Part model, mm, in its own coordinate system. Face numbers are marked on the shaded views. A direction names the side the tool comes from. Coordinates: 2 decimals unless noted, no trailing zeros. Order: outer loops, then holes, each group sorted by start corner. A loop starts at its lowest first (then second) coordinate and runs counter-clockwise, first axis right, second up.
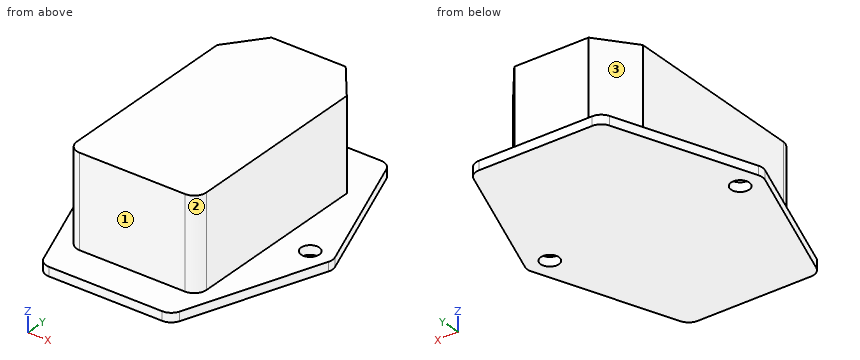
```python
from build123d import *

# Parameters (mm, degrees)
BOSS_EXTRUDE1_DEPTH     = 19.05
BOSS_EXTRUDE2_DEPTH     = 1.8796
CUT_EXTRUDE1_DEPTH      = 22.606
CUT_EXTRUDE1_DEPTH_BACK = 20.4216
SKETCH6_R               = 1.905


with BuildPart() as part:
    # Sketch1 → Boss-Extrude1 (new body)
    with BuildSketch(Plane.XY):
        with BuildLine():
            Line((2.54, 0), (24.5618, 0))
            ThreePointArc((24.5618, 0), (26.357851224, 0.743948776), (27.1018, 2.54))
            Line((27.1018, 2.54), (27.1018, 41.4401))
            Line((27.1018, 41.4401), (21.3106, 48.809471297))
            Line((21.3106, 48.809471297), (5.7912, 48.809471297))
            Line((5.7912, 48.809471297), (0, 41.4401))
            Line((0, 41.4401), (0, 2.54))
            ThreePointArc((0, 2.54), (0.743948776, 0.743948776), (2.54, 0))
        make_face()
    extrude(amount=BOSS_EXTRUDE1_DEPTH)

    # Sketch2 → Boss-Extrude2 (add)
    with BuildSketch(Plane.XY):
        with BuildLine():
            Line((1.657581985, 53.267171297), (25.317218015, 53.267171297))
            ThreePointArc((25.317218015, 53.267171297), (26.770442849, 52.81037498), (27.700968665, 51.604287506))
            Line((27.700968665, 51.604287506), (37.914530402, 23.846751857))
            ThreePointArc((37.914530402, 23.846751857), (38.070779753, 22.969635649), (37.914530402, 22.09251944))
            Line((37.914530402, 22.09251944), (27.700968665, -5.665016208))
            ThreePointArc((27.700968665, -5.665016208), (26.770442849, -6.871103683), (25.317218015, -7.3279))
            Line((25.317218015, -7.3279), (1.657581985, -7.3279))
            ThreePointArc((1.657581985, -7.3279), (0.204357151, -6.871103683), (-0.726168665, -5.665016208))
            Line((-0.726168665, -5.665016208), (-10.939730402, 22.09251944))
            ThreePointArc((-10.939730402, 22.09251944), (-11.095979753, 22.969635649), (-10.939730402, 23.846751857))
            Line((-10.939730402, 23.846751857), (-0.726168665, 51.604287506))
            ThreePointArc((-0.726168665, 51.604287506), (0.204357151, 52.81037498), (1.657581985, 53.267171297))
        make_face()
    extrude(amount=-BOSS_EXTRUDE2_DEPTH)

    # Sketch6 → Cut-Extrude1 (cut, two sides: drawn at the far end of the back side and taken through both)
    with BuildSketch(Plane.XY.offset(-CUT_EXTRUDE1_DEPTH_BACK)):
        with Locations(Location((33.384479753, 22.969635649, 0), (0, 0, 180))):
            Circle(SKETCH6_R)
        with Locations(Location((-6.409679753, 22.969635649, 0), (0, 0, 180))):
            Circle(SKETCH6_R)
    extrude(amount=CUT_EXTRUDE1_DEPTH + CUT_EXTRUDE1_DEPTH_BACK, mode=Mode.SUBTRACT)


solid = part.part
```
(1) Tool access for the marked faces 1, 2 and 3: list every direction of +Z, -Z, +X, -X, +Y, -Y with a clear straight run to the whole face (end or side of a thin tool).
(2) Drop flat-ended pins along their axis: pin 1 (4 mm diameter, centred on x = -2.5, y = 37, fed in from +Z); pin 2 (9.5 mm diameter, centred on y = 27, z = 6.5, fed in from +X); pin 3 (2.5 mm diameter, centred on x = 33.38, y = 22.97, fed in from +Z); pin 4 (5 mm diameter, centred on x = 22.5, z = 1, fed in from -Y). Give the stop position or say it passes through.
(3) Slice it at C-C, the plane x = -3. Give the cut face in (y, z).
(4) Slice it at A-A, the plane z = 1.75. Give the cut face in (x, y), then the cut area to 3 significant figures.
(5) Slice it at B-B, the plane y = 45.5. Give the cut face in (x, z), then the cut area to 3 significant figures.
(6) Probe line 1 (X direction, y = 34, z = 11.25); line 2 (Z direction, x = -2.5, y = 12); line 3 (Y direction, x = 17, z = 18). List the from-to ranges inside material, lowest first.
Here are the results:
1. face 1: +Z, +X, -X, -Y
1. face 2: +Z, +X, -Y
1. face 3: +Z, -X, +Y
2. pin 1: stops at z = 0
2. pin 2: stops at x = 27.1
2. pin 3: passes through
2. pin 4: stops at y = -7.33
3. outline: (0.51, -1.88) - (45.42, -1.88) - (45.42, 0) - (0.51, 0) - close
4. outline: (0, 2.54) arc R2.54 ccw to (2.54, 0) - (24.56, 0) arc R2.54 ccw to (27.1, 2.54) - (27.1, 41.44) - (21.31, 48.81) - (5.79, 48.81) - (0, 41.44) - close
4. area: 1,280 mm2
5. outline: (-2.97, -1.88) - (29.95, -1.88) - (29.95, 0) - (23.91, 0) - (23.91, 19.05) - (3.19, 19.05) - (3.19, 0) - (-2.97, 0) - close
5. area: 457 mm2
6. line 1: x = 0 to 27.1
6. line 2: z = -1.88 to 0
6. line 3: y = 0 to 48.81
